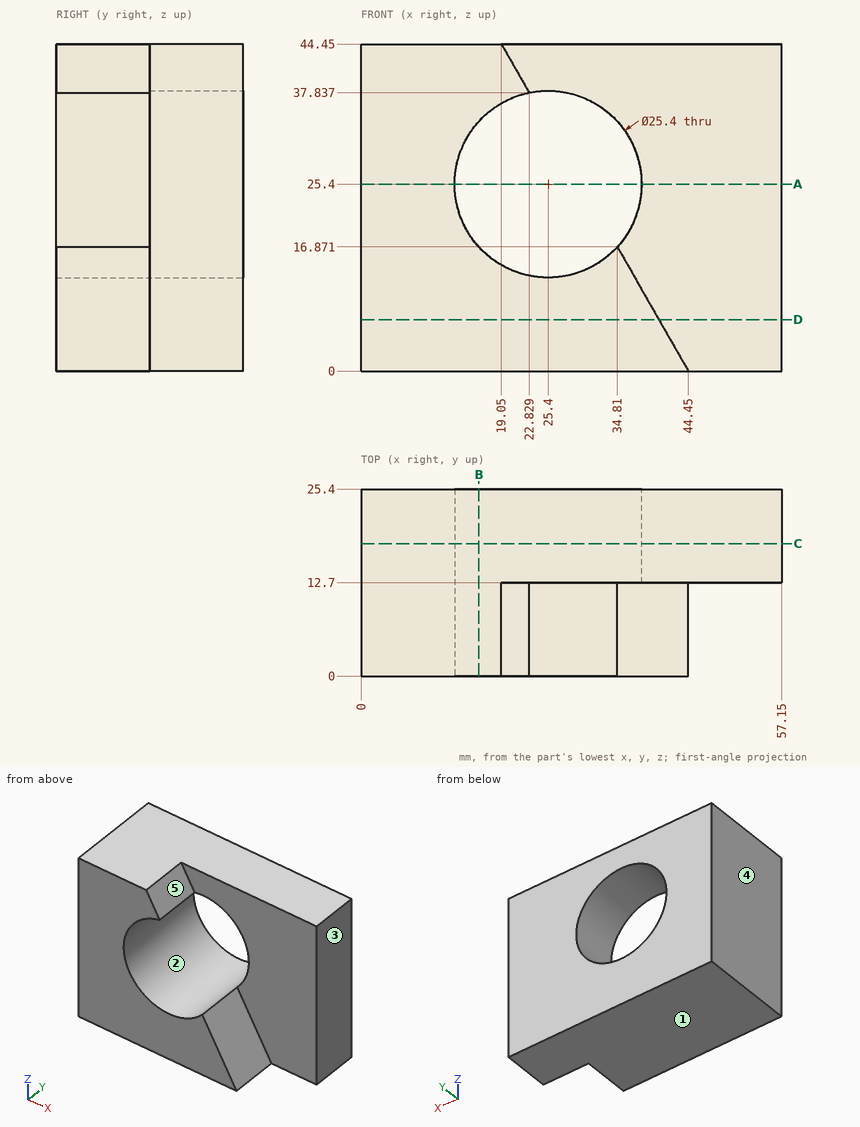
Source: three-view drawing plus pictorial views. Frame: mm from the lowest corner of the part. A direction names the side the tool comes from. Give positions to 0.01 mm unless a question says otherwise; leave off trailing zeros. Order: outer loops, then holes, each group sorted by start corner. A loop starts at its lowest first (then second) coordinate and runs counter-clockwise, first axis right, second up. Notation, with made-up numbers: M -8.5,54.5 L 29.5,54.5 A34 ccw 29.5,88.5 Z; hole C 7,-21.5 d9. An arc over 180 degrees is marked long. One line per question, with ' | ' between items.
1) Contact query for flat-ended pins moving along their axis: P1, Ø6, axis at y = 5, z = 6.5, coming from the +X side; P2, Ø1.5, axis at y = 3, z = 26, coming from the +X side; P3, Ø15, axis at x = 25.4, z = 25.4, coming from the -Y side. Output: stop coordinate, or through.
Filled in:
P1: stops at x = 42.45 | P2: stops at x = 12.77 | P3: passes through
2) Section A-A on z = 25.4. Output: boundary loops of the cut face in (x, y).
Filled in:
outline: M 0,0 L 12.7,0 L 12.7,25.4 L 0,25.4 Z; M 38.1,12.7 L 57.15,12.7 L 57.15,25.4 L 38.1,25.4 Z
3) Ray query, L1, parallel to Z at x = 25.4, y = 18.25; L2, parallel to X at y = 16, z = 32.5; L3, parallel to Z at x = 16, y = 19. Return the intervals inside material, ascending.
Filled in:
L1: z = 0 to 12.7, 38.1 to 44.45 | L2: x = 0 to 14.87, 35.93 to 57.15 | L3: z = 0 to 16.86, 33.94 to 44.45
4) Section B-B on x = 16. Output: boundary loops of the cut face in (y, z), and give its area (3 significant figures).
Filled in:
outline: M 0,0 L 25.4,0 L 25.4,16.86 L 0,16.86 Z; M 0,33.94 L 25.4,33.94 L 25.4,44.45 L 0,44.45 Z | area: 695 mm2
5) Draft query along X for the marked faces 1, 2 and 3. Return one class per face: pulls with the +X half, pulls with the -X half, needs draft (parallel to the pull), parting line crosses it, or undercut.
Filled in:
face 1: needs draft | face 2: undercut | face 3: pulls with the +X half
6) Section C-C on y = 18. Output: boundary loops of the cut face in (x, z), and give its area (3 significant figures).
Filled in:
outline: M 0,0 L 57.15,0 L 57.15,44.45 L 0,44.45 Z; hole C 25.4,25.4 d25.4 | area: 2,030 mm2
7) Access query for the marked faces 4 and 5. Directions: +Z, -Z, +X, -X, +Y, -Y. A direction counts if a zero-diameter tool reaches every point of the face in a straight line with its end or side. Return the directions, or none.
Filled in:
face 4: +Z, -Z, -X, +Y, -Y | face 5: +Z, +X, -Y
8) Section D-D on z = 7. Output: boundary loops of the cut face in (x, y), and give its area (3 significant figures).
Filled in:
outline: M 0,0 L 40.45,0 L 40.45,12.7 L 57.15,12.7 L 57.15,25.4 L 0,25.4 Z | area: 1,240 mm2
